```python
from build123d import *

# Parameters (mm, degrees)
MODEL_R             = 1.298950001
MODEL_R_2           = 1.499950004
BOSS_EXTRUDE1_DEPTH = 3


with BuildPart() as part:
    # Model → Boss-Extrude1 (new body)
    with BuildSketch(Plane.XY):
        with BuildLine():
            Line((72.2662, 46.25), (72.2662, 56.421043711))
            ThreePointArc((72.2662, 56.421043711), (71.145459643, 58.637903109), (68.738, 59.25))
            Line((68.738, 59.25), (51.7943, 59.25))
            ThreePointArc((51.7943, 59.25), (49.381832487, 58.63325007), (48.2662, 56.4071))
            Line((48.2662, 56.4071), (48.2662, 46.25))
            Line((48.2662, 46.25), (48.2662, 19.75))
            ThreePointArc((48.2662, 19.75), (49.144899998, 17.628699998), (51.2662, 16.75))
            Line((51.2662, 16.75), (69.2662, 16.75))
            ThreePointArc((69.2662, 16.75), (71.387450001, 17.628749999), (72.2662, 19.75))
            Line((72.2662, 19.75), (72.2662, 46.25))
        make_face()
        with Locations((51.76615, 56.45005)):
            Circle(MODEL_R, mode=Mode.SUBTRACT)
        with Locations((68.76615, 56.45005)):
            Circle(MODEL_R, mode=Mode.SUBTRACT)
        with Locations((51.76615, 29.25005)):
            Circle(MODEL_R, mode=Mode.SUBTRACT)
        with Locations((68.76615, 29.25005)):
            Circle(MODEL_R, mode=Mode.SUBTRACT)
        with Locations((51.216249997, 19.750049997)):
            Circle(MODEL_R_2, mode=Mode.SUBTRACT)
        with Locations((69.316249997, 19.750049997)):
            Circle(MODEL_R_2, mode=Mode.SUBTRACT)
        Polygon((69.2662, 48.75), (69.2662, 36.75), (66.2662, 36.75), (66.2662, 31.25), (54.2662, 31.25), (54.2662, 36.75), (51.2662, 36.75), (51.2662, 48.75), (54.2662, 48.75), (54.2662, 54.25), (66.2662, 54.25), (66.2662, 48.75), align=None, mode=Mode.SUBTRACT)
    extrude(amount=BOSS_EXTRUDE1_DEPTH)


solid = part.part
```
Geometry: final body of the model. Coordinates: model frame, mm. A direction names the side the tool comes from. Round coordinates to 2 decimals unless told otherwise and drop trailing zeros. Order: outer loops, then holes, each group sorted by start corner. A loop starts at its lowest first (then second) coordinate and runs counter-clockwise, first axis right, second up. Notation, with made-up numbers: (-24.5, -10) -> (33.5, -10) arc R13 cw to (33.5, 1) -> close; hole circle Ø1 at (-1.5, 80). An arc over 180 degrees is marked (long way). Use one line per item in the form item = value. Start each with the question number.
1. Cut plane A-A (x = 66.75). Return the cut outline in (y, z), then the cut area to 3 significant figures.
2. Line query: probe 1 along X at (y, z) = (34, 1.5); probe 2 along X at (y, z) = (19, 2.85); probe 3 along Y at (x, z) = (62, 0.95). Output: solid intervals per line, ascending.
3. Reachability of faces 1 (the face through (60, 59.25, 1)), 2 (the face through (71.364, 17.606, 1.479)), 3 (the face through (60, 54.25, 1)) from +Z, -Z, +X, -X, +Y, -Y: full face, straight path, thin tool, end or side. Return the list, or none.
4. Cut plane B-B (y = 51.5). Return the cut outline in (x, z), then the cut area to 3 significant figures.
5. Cut plane C-C (z = 2.4). Return the cut outline in (x, y), then the cut area to 3 significant figures.
6. Pin query (flat end, axial travel): pin 1 Ø1.5 at (x, z) = (53, 2) entering from +Y; pin 2 Ø2.5 at (x, y) = (51.22, 19.75) entering from +Z. Return the tip coordinate at first contact, or that it passes through.
Solution:
q1.outline = (16.75, 0) -> (36.75, 0) -> (36.75, 3) -> (16.75, 3) -> close; (48.75, 0) -> (59.25, 0) -> (59.25, 3) -> (48.75, 3) -> close
q1.area = 91.5 mm^2
q2.probe_1 = 48.27 to 54.27, 66.27 to 72.27
q2.probe_2 = 48.36 to 49.92, 52.52 to 68.02, 70.62 to 72.17
q2.probe_3 = 16.75 to 31.25, 54.25 to 59.25
q3.face_1 = +Z, -Z, +Y
q3.face_2 = +Z, -Z, +X, -Y
q3.face_3 = +Z, -Z
q4.outline = (48.27, 0) -> (54.27, 0) -> (54.27, 3) -> (48.27, 3) -> close; (66.27, 0) -> (72.27, 0) -> (72.27, 3) -> (66.27, 3) -> close
q4.area = 36.0 mm^2
q5.outline = (48.27, 19.75) arc R3 ccw to (51.27, 16.75) -> (69.27, 16.75) arc R3 ccw to (72.27, 19.75) -> (72.27, 56.42) arc R3 ccw to (68.74, 59.25) -> (51.79, 59.25) arc R3 ccw to (48.27, 56.41) -> close; hole circle Ø3 at (51.22, 19.75); hole circle Ø2.6 at (51.77, 29.25); hole circle Ø2.6 at (51.77, 56.45); hole (51.27, 36.75) -> (54.27, 36.75) -> (54.27, 31.25) -> (66.27, 31.25) -> (66.27, 36.75) -> (69.27, 36.75) -> (69.27, 48.75) -> (66.27, 48.75) -> (66.27, 54.25) -> (54.27, 54.25) -> (54.27, 48.75) -> (51.27, 48.75) -> close; hole circle Ø2.6 at (68.77, 29.25); hole circle Ø2.6 at (68.77, 56.45); hole circle Ø3 at (69.32, 19.75)
q5.area = 629 mm^2
q6.pin_1 = 59.25
q6.pin_2 = through
